```python
from build123d import *

# Parameters (mm, degrees)
F1_DEPTH = 1000


with BuildPart() as f1:
    # F0 (on Top) → F1 (new body)
    with BuildSketch(Plane.XY):
        with BuildLine():
            Line((125.716477, 120), (-136.783523, 120))
            Line((-136.783523, 120), (-136.783523, -180))
            Line((-136.783523, -180), (1.716477, -180))
            ThreePointArc((1.716477, -180), (18.335515, -120), (1.716477, -60))
            ThreePointArc((1.716477, -60), (7.574341, -45.857864), (21.716477, -40))
            Line((21.716477, -40), (21.716477, -30))
            ThreePointArc((21.716477, -30), (42.92968, -21.213203), (51.716477, 0))
            Line((51.716477, 0), (51.716477, 5))
            Line((51.716477, 5), (56.716477, 5))
            ThreePointArc((56.716477, 5), (60.252011, 3.535534), (61.716477, 0))
            Line((61.716477, 0), (71.716477, 0))
            Line((71.716477, 0), (71.716477, 35))
            Line((71.716477, 35), (77.716477, 35))
            ThreePointArc((77.716477, 35), (79.66063, 40.924807), (84.737143, 44.545867))
            ThreePointArc((84.737143, 44.545867), (90.074672, 48.539274), (91.716477, 55))
            Line((91.716477, 55), (97.716477, 55))
            Line((97.716477, 55), (97.716477, 65))
            ThreePointArc((97.716477, 65), (105.346334, 73.838605), (105.718453, 85.508959))
            ThreePointArc((105.718453, 85.508959), (109.315655, 102.446682), (125.716477, 108))
            Line((125.716477, 108), (125.716477, 120))
        make_face()
    extrude(amount=F1_DEPTH)


solid = f1.part
```
The model under review builds one solid part; all positions refer to its coordinate system, in mm. A direction names the side the tool comes from. Round coordinates to 2 decimals unless told otherwise and drop trailing zeros. Write each loop counter-clockwise with the first axis right and the second up, starting at its lowest first coordinate (ties: lowest second). Pieces come first, ordered by that corner, then holes. Notation, with made-up numbers: M 35.5,-11.75 L 89.5,-11.75 A20 ccw 89.5,22.25 Z; hole C 23.25,28 d4. An arc over 180 degrees is marked long. Use CSV: the item, a comma, the result in double quotes. Start each with the question number.
(1) The part is to be moulded in two halves that separate along Y. For faces 4 (the face through (18.332, -120.882, 493)), 5 (the face through (-69, -180, 493)), 6 (the face through (-37, 5, 0)), say which applies: +Y half, -Y half, draft (parallel to the pull), parting line (faces both ways), or undercut.
(2) We need section B-B, the plane y = -97.5. State the section outline as (x, z) points.
(3) Tool access review of faces 1 (the face through (71.716, 17, 493)), 2 (the face through (-4, 120, 493)), 3 (the face through (7.42, -46.014, 493)): name each direction out of +Z, -Z, +X, -X, +Y, -Y from which nothing blocks a thin tool from reaching the whole face with its end or side.
(4) Clearance check with flat-ended pins moving along their axes: P1, Ø4, axis at y = 3, z = 622, coming from the +X side; P2, Ø1.8, axis at x = 74, z = 417, coming from the -Y side; P3, Ø1.5, axis at x = 68, z = 603.5, coming from the -Y side. State where each tip first meets the part, or that it passes through.
(5) We need section C-C, the plane x = 38.5. State the section outline as (y, z) points.
(6) We need section A-A, the plane z = 785. State the section outline as (x, y) points.
(7) For line 1 along X through (y, z) = (101.5, 648); line 2 along X through (y, z) = (3.5, 686.5); line 3 along Y through (x, z) = (114.5, 344.5), list the stretches that pass through material, from the lowest coordinate up.
Findings:
1,face 4,"undercut"
1,face 5,"-Y half"
1,face 6,"draft"
2,outline,"M -136.78,0 L 16.14,0 L 16.14,1000 L -136.78,1000 Z"
3,face 1,"+Z, -Z, +X, -Y"
3,face 2,"+Z, -Z, +X, -X, +Y"
3,face 3,"+Z, -Z, +X"
4,P1,"x = 71.72"
4,P2,"y = 35"
4,P3,"y = 0"
5,outline,"M -24.87,0 L 120,0 L 120,1000 L -24.87,1000 Z"
6,outline,"M -136.78,-180 L 1.72,-180 A116.62 ccw 1.72,-60 A20 cw 21.72,-40 L 21.72,-30 A30 ccw 51.72,0 L 51.72,5 L 56.72,5 A5 cw 61.72,0 L 71.72,0 L 71.72,35 L 77.72,35 A10 cw 84.74,44.55 A10 ccw 91.72,55 L 97.72,55 L 97.72,65 A17.5 ccw 105.72,85.51 A17.5 cw 125.72,108 L 125.72,120 L -136.78,120 Z"
7,line 1,"-136.78 to 108.53"
7,line 2,"-136.78 to 51.72, 60.29 to 71.72"
7,line 3,"106.44 to 120"
